Geometry: final body of the model. Coordinates: model frame, mm. Face numbers are marked on the shaded views. A direction names the side the tool comes from. Give positions to 0.01 mm unless a question says otherwise; leave off trailing zeros. Write each loop counter-clockwise with the first axis right and the second up, starting at its lowest first coordinate (ties: lowest second). Pieces come first, ordered by that corner, then holes. Notation, with made-up numbers: (-3.75, 34) - (32.25, 34) arc R27 cw to (32.25, 52) - close; hole circle Ø8 at (69, 54.5). An arc over 180 degrees is marked (long way). Return JSON: item names as keys, results as strings.
from build123d import *

# Parameters (mm, degrees)
BOSS_EXTRUDE1_DEPTH        = 21
SKETCH2_W                  = 38
SKETCH2_H                  = 23
BOSS_EXTRUDE2_DEPTH        = 52
BOSS_EXTRUDE3_DEPTH        = 26
CHAMFER1_SIZE              = 1
M12_TAPPED_HOLE1_D         = 10.2
M12_TAPPED_HOLE1_DEPTH     = 23
F_12_0_12_DIAMETER_HOLE1_D = 12
CHAMFER2_SIZE              = 1


with BuildPart() as part:
    # Sketch1 → Boss-Extrude1 (new body)
    with BuildSketch(Plane.XY):
        Polygon((-19, 0), (19, 0), (19, -23), (18, -23), (18, -25), (55, -62), (55, -88), (-55, -88), (-55, -62), (-18, -25), (-18, -23), (-19, -23), align=None)
    extrude(amount=BOSS_EXTRUDE1_DEPTH)

    # Sketch2 → Boss-Extrude2 (add)
    with BuildSketch(Plane(origin=(0, 0, 0), x_dir=(-1, 0, 0), z_dir=(0, 0, -1))):
        with Locations((0, -11.5)):
            Rectangle(SKETCH2_W, SKETCH2_H)
    extrude(amount=-BOSS_EXTRUDE2_DEPTH)

    # Sketch3 → Boss-Extrude3 (add)
    with BuildSketch(Plane.XY.offset(21)):
        Polygon((-7, -50), (7, -50), (28, -71), (28, -88), (-28, -88), (-28, -71), align=None)
    extrude(amount=BOSS_EXTRUDE3_DEPTH)

    # Chamfer1
    chamfer1_edges = [part.edges().sort_by_distance(p)[0] for p in [
        (0, -23, 52),
        (-19, -23, 26),
        (-19, -11.5, 52),
        (19, -23, 26),
        (19, -11.5, 52),
        (19, 0, 26),
        (0, 0, 52),
        (-19, 0, 26),
    ]]
    chamfer(chamfer1_edges, length=CHAMFER1_SIZE)

    # M12 Tapped Hole1
    with Locations(Plane(origin=(0, 0, 0), x_dir=(1, 0, 0), z_dir=(0, 1, 0))):
        with Locations((0, -37)):
            Hole(M12_TAPPED_HOLE1_D / 2, depth=M12_TAPPED_HOLE1_DEPTH)

    # Ø12.0 (12) Diameter Hole1 (through all)
    with Locations(Plane.XY.offset(21)):
        with Locations((-13.5, -42), (13.5, -42)):
            Hole(F_12_0_12_DIAMETER_HOLE1_D / 2)

    # Chamfer2
    chamfer2_edges = [part.edges().sort_by_distance(p)[0] for p in [
        (7, -50, 34),
        (-7, -50, 34),
    ]]
    chamfer(chamfer2_edges, length=CHAMFER2_SIZE)


solid = part.part
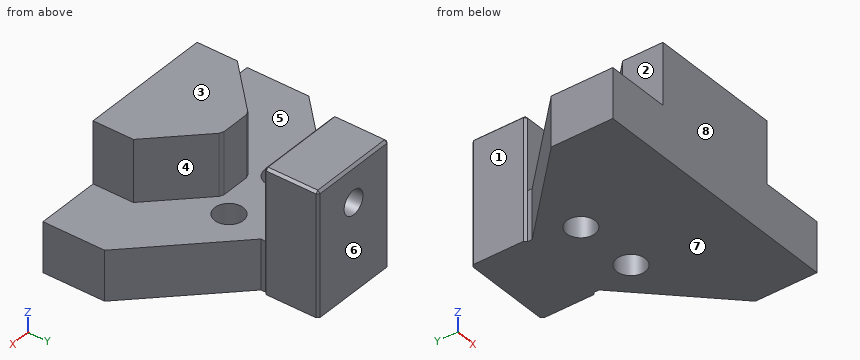
Q1. Section query B-B, the plane x = -13.5. Return the cut outline in (y, z), plus the area to 3 significant figures.
Answer key:
{"outline": "(-88, 0) - (-48, 0) - (-48, 21) - (-56.5, 21) - (-56.5, 47) - (-88, 47) - close; (-36, 0) - (0, 0) - (0, 51) - (-1, 52) - (-22, 52) - (-23, 51) - (-23, 21) - (-36, 21) - close", "area": "3,130 mm^2"}
Q2. Pin query (flat end, axial travel): P1, Ø18.5, axis at y = -82, z = 31.5, coming from the -X side; P2, Ø2, axis at x = 22.5, z = 40.5, coming from the +Y side; P3, Ø1, axis at y = -24, z = 11, coming from the -X side; P4, Ø19, axis at x = -13.5, y = -42, coming from the -Z side. Return the tip coordinate at first contact, or that it passes through.
Answer key:
{"P1": "stops at x = -28", "P2": "stops at y = -64.5", "P3": "stops at x = -18", "P4": "stops at z = 0"}
Q3. Section query C-C, the plane y = -42. Return the cut outline in (x, z).
Answer key:
{"outline": "(-35, 0) - (-19.5, 0) - (-19.5, 21) - (-35, 21) - close; (-7.5, 0) - (7.5, 0) - (7.5, 21) - (-7.5, 21) - close; (19.5, 0) - (35, 0) - (35, 21) - (19.5, 21) - close"}
Q4. Mould query, pull axis Y, two halves, no side actions, for the marked faces 5, 6, 7 and 8. Classes: pulls with the +Y half, pulls with the -Y half, needs draft (parallel to the pull), parting line crosses it, or undercut.
Answer key:
{"face 5": "undercut", "face 6": "pulls with the +Y half", "face 7": "needs draft", "face 8": "pulls with the -Y half"}
Q5. Section query D-D, the plane z = 37. Return the cut outline in (x, y).
Answer key:
{"outline": "(-28, -88) - (28, -88) - (28, -71) - (7.71, -50.71) - (6, -50) - (-6, -50) - (-7.71, -50.71) - (-28, -71) - close; (-19, -22) - (-18, -23) - (-5.1, -23) - (-5.1, 0) - (-18, 0) - (-19, -1) - close; (5.1, -23) - (18, -23) - (19, -22) - (19, -1) - (18, 0) - (5.1, 0) - close"}
Q6. Set-up query: the marked faces 1, 2, 3 and 4. Return all of +Z, -Z, +X, -X, +Y, -Y with unobstructed straight access to the full face (end or side cutting, diameter ignored); none if empty.
Answer key:
{"face 1": "+Z, -Z, -X, +Y", "face 2": "+Z, -X, +Y, -Y", "face 3": "+Z, +X, -X, -Y", "face 4": "+Z, +X"}
Q7. Section query A-A, the plane z = 23. Return the cut outline in (x, y), plus the area to 3 significant figures.
Answer key:
{"outline": "(-28, -88) - (28, -88) - (28, -71) - (7.71, -50.71) - (6, -50) - (-6, -50) - (-7.71, -50.71) - (-28, -71) - close; (-19, -22) - (-18, -23) - (18, -23) - (19, -22) - (19, -1) - (18, 0) - (-18, 0) - (-19, -1) - close", "area": "2,560 mm^2"}
Q8. Material intervals for probe 1 along Z at (x, y) = (0, -17.5); probe 2 along Y at (x, z) = (13, 13); probe 3 along X at (y, z) = (-14.25, 37), sorted ascending. Write a range as [from, to].
Answer key:
{"probe 1": "z = [0, 31.9], [42.1, 52]", "probe 2": "y = [-88, -47.98], [-36.02, 0]", "probe 3": "x = [-19, -5.1], [5.1, 19]"}
